The listing builds one solid part. Answer for the finished solid, in the listing's coordinates (mm). Give positions to 0.01 mm unless a question says otherwise; leave off trailing zeros. Order: outer loops, then holes, each group sorted by start corner. A loop starts at its lowest first (then second) coordinate and runs counter-clockwise, first axis right, second up. Notation, with made-up numbers: (-28, 78) - (22, 78) arc R25 cw to (22, 111) - close; hole circle Ø6 at (-2, -4.75). An arc over 180 degrees is marked (long way). Use CSV: the item, a comma, the result in double quotes.
Autodesk Inventor part; units mm, degrees
ref_plane "YZ Plane" through (0, 0, 0) normal (1, 0, 0) x (0, 1, 0)
ref_plane "XZ Plane" through (0, 0, 0) normal (0, 1, 0) x (-1, 0, 0)
ref_plane "XY Plane" through (0, 0, 0) normal (0, 0, 1) x (1, 0, 0)
sketch "Sketch1" plane through (0, 0, 0) normal (0, 1, 0) x (-1, 0, 0)
  line L0 (70, 105) -> (-70, 105)
  line L1 (-70, 105) -> (-70, -105)
  line L2 (-70, -105) -> (70, -105)
  line L3 (70, -105) -> (70, 105)
  line L4 (70, 105) -> (-70, -105) construction
  point P0 (0, 0)
  point P1 (0, 0)
  dimension "d0" = 140
  dimension "d1" = 210
extrude "Plate1" add sketch "Sketch1" along normal blind 3
fillet "Corner Round1" radius 6 3 edges at (70, 1.5, 105) (-70, 1.5, 105) (-70, 1.5, -105)
chamfer "Corner Chamfer1" distance 27 angle 50.38 1 edges at (70, 1.5, -105) measured on face at (25.3333, 1, -105)
equation "\"d2\" = Thickness"
equation "\"BendReliefWidth\" = Thickness"
equation "\"BendReliefDepth\" = 0.5 * Thickness"
equation "\"CornerReliefSize\" = 4 * Thickness"
equation "\"MinimumRemnant\" = 2 * Thickness"
equation "\"TransitionRadius\" = BendRadius"
equation "\"JacobiRadiusSize\" = BendRadius"
equation "\"GapSize\" = Thickness"
properties part number "MSC 909 TUBE SUPPORT 3" material "Stainless Steel"
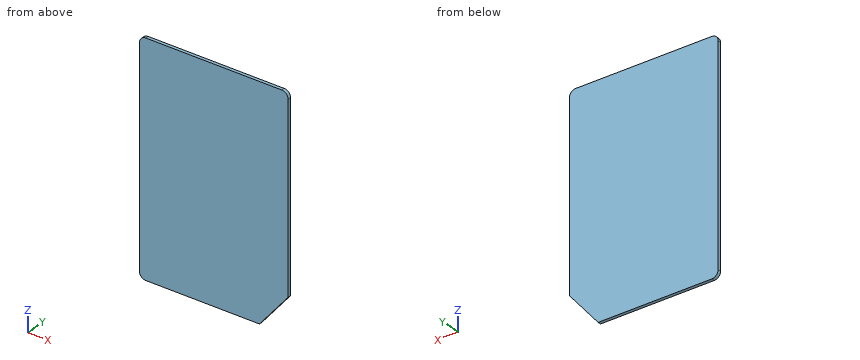
Item 1: Find the intervals of material crossed by line 1 along Z through (x, y) = (61, 2.5); line 2 along Z through (x, y) = (52.5, 2.85); line 3 along X through (y, z) = (0.45, -82.5), in increasing order.
Taken from the geometry:
line 1,"-83.26 to 105"
line 2,"-93.52 to 105"
line 3,"-70 to 61.63"
Item 2: The part is cut by section A-A (y = 0.6). Give the vertices of the cut face in (x, z), and give its area (3 significant figures).
Taken from the geometry:
outline,"(-70, -99) arc R6 ccw to (-64, -105) - (43, -105) - (70, -72.39) - (70, 99) arc R6 ccw to (64, 105) - (-64, 105) arc R6 ccw to (-70, 99) - close"
area,"28,900 mm^2"
Item 3: The part is cut by section B-B (z = -75). Give the vertices of the cut face in (x, y).
Taken from the geometry:
outline,"(-70, 0) - (67.84, 0) - (67.84, 3) - (-70, 3) - close"
